Can you work these out from the model? Positions are in its coordinate system, mm. A direction names the side the tool comes from. Give positions to 0.01 mm unless a question says otherwise; leave off trailing zeros. Order: outer loops, then holes, each group sorted by start corner. A loop starts at its lowest first (then second) coordinate and runs counter-clockwise, first axis right, second up. Notation, with made-up numbers: M 49.5,33.25 L 72.5,33.25 A34 cw 72.5,63.25 Z; hole C -9.5,58.5 d3. An arc over 180 degrees is marked long. Write each question's results on one line, items separated by ' | '.
Autodesk Inventor part; units mm, degrees
ref_plane "YZ Plane" through (0, 0, 0) normal (1, 0, 0) x (0, 1, 0)
ref_plane "XZ Plane" through (0, 0, 0) normal (0, 1, 0) x (-1, 0, 0)
ref_plane "XY Plane" through (0, 0, 0) normal (0, 0, 1) x (1, 0, 0)
sketch "Sketch1" plane through (0, 0, 0) normal (0, 1, 0) x (-1, 0, 0)
  circle A0 centre (0, 0) radius 16.256
  dimension "d0" = 32.512
extrude "Extrusion1" add sketch "Sketch1" along normal blind 5
sketch "Sketch11" plane through (0, 5, 0) normal (0, 1, 0) x (1, 0, 0)
  circle A0 centre (0, 0) radius 12.7
  dimension "d38" = 25.4
extrude "Extrusion6" add sketch "Sketch11" along normal blind 11.4
sketch "Sketch12" plane through (0, 16.4, 0) normal (0, 1, 0) x (1, 0, 0)
  circle A0 centre (0, 0) radius 16.256
  dimension "d41" = 32.512
extrude "Extrusion7" add sketch "Sketch12" along normal blind 13.85
sketch "Sketch13" plane through (0, 30.25, 0) normal (0, 1, 0) x (1, 0, 0)
  point P0 (0, 0)
  point P1 (0, 0)
hole "Hole2" at (0, 30.25, 0) direction (0, -1, 0) diameter 6 depth 6 tip angle 118
thread "Thread3"
sketch "Sketch14" plane through (0, 0, 0) normal (0, -1, 0) x (1, 0, 0)
  circle A0 centre (0, 0) radius 3
hole "Hole3" at (0, 0, 0) direction (0, 1, 0) diameter 6 depth 6 tip angle 118
thread "Thread4"
properties part number "POSTE_ESPEJO"
(1) Will these pins go through, and if not, where does the flat tip stop? P1, Ø3, axis at x = 1, z = 6.5, coming from the -Y side; P2, Ø4, axis at y = 24, z = 11.5, coming from the +X side; P3, Ø6, axis at y = 15, z = 12.5, coming from the +X side; P4, Ø1.5, axis at x = 9, y = 21, coming from the +Z side.
Data:
P1: stops at y = 0 | P2: stops at x = 13.19 | P3: stops at x = 12.93 | P4: stops at z = 14.01
(2) Imagine slicing it at B-B, the plane y = 17.5. Write out the boundary of the cut face in (x, z), plus the area to 3 significant figures.
Data:
outline: C 0,0 d32.51 | area: 830 mm2
(3) I need wall thicknesses on L1, parallel to Z at x = 0, y = 3; L2, parallel to Y at x = 12, z = 8. Which ranges of each line are inside material? Lowest first, please. Write a range as from..to.
Data:
L1: z = -16.26..-3, 3..16.26 | L2: y = 0..5, 16.4..30.25
(4) For faces 4 (the face through (0, 27, -3)), 5 (the face through (0.2, 0, -3.4)), 6 (the face through (0, 3, 3)), 7 (the face through (-7, 5, -11)), 8 (the face through (-3.52, 23.23, -15.87)), which set-ups out of +Z, -Z, +X, -X, +Y, -Y let a thin tool reach every point of the face, with its end or its side?
Data:
face 4: +Y | face 5: +Z, -Z, +X, -X, -Y | face 6: -Y | face 7: none | face 8: +Y, -Y
(5) Imagine slicing it at C-C, the plane z = -5. Write out the boundary of the cut face in (x, y).
Data:
outline: M -15.47,0 L 15.47,0 L 15.47,5 L 11.67,5 L 11.67,16.4 L 15.47,16.4 L 15.47,30.25 L -15.47,30.25 L -15.47,16.4 L -11.67,16.4 L -11.67,5 L -15.47,5 Z
(6) Imagine slicing it at A-A, the plane z = -12. Write out the boundary of the cut face in (x, y).
Data:
outline: M -10.97,0 L 10.97,0 L 10.97,5 L 4.16,5 L 4.16,16.4 L 10.97,16.4 L 10.97,30.25 L -10.97,30.25 L -10.97,16.4 L -4.16,16.4 L -4.16,5 L -10.97,5 Z
(7) We'd pull the mould along Z, two halves only. Please class faces 1 (the face through (-0.2, 30.25, 3.4)), 2 (the face through (0.156, 22.76, 0.497)), 3 (the face through (-2.75, 10.62, -12.4)): +Z half, -Z half, draft (parallel to the pull), parting line (faces both ways), or undercut.
Data:
face 1: draft | face 2: undercut | face 3: parting line
